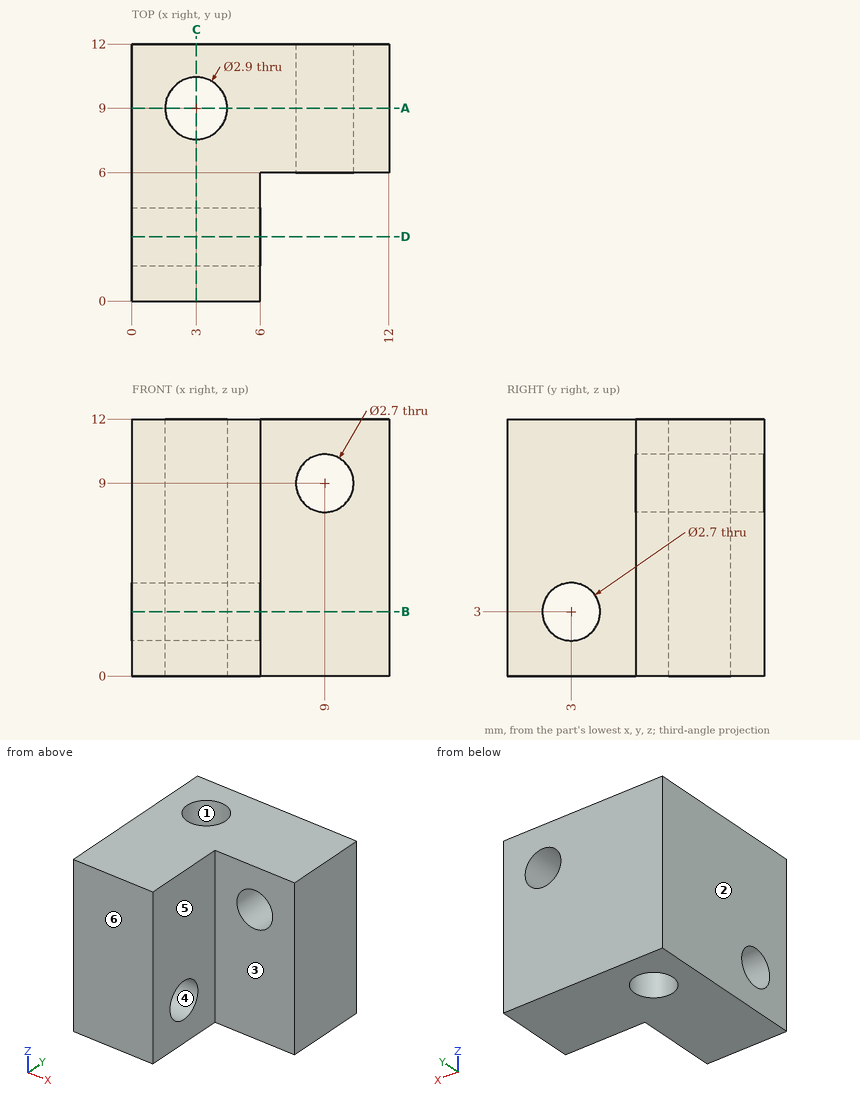
Geometry: see drawing. Coordinates: mm, zero at the bounding-box minimum. A direction names the side the tool comes from. Give positions to 0.01 mm unless a question says otherwise; leave off trailing zeros. Order: outer loops, then holes, each group sorted by start corner. A loop starts at its lowest first (then second) coordinate and runs counter-clockwise, first axis right, second up. Notation, with made-up numbers: (4.5, 77) -> (24.5, 77) arc R14 cw to (24.5, 99) -> close; hole circle Ø11 at (18, 4.5). An arc over 180 degrees is marked (long way). Write each question's results on one line, items separated by ' | '.
1) Cut plane A-A (y = 9). Output: boundary loops of the cut face in (x, z).
Geometry says:
outline: (0, 0) -> (1.55, 0) -> (1.55, 12) -> (0, 12) -> close; (4.45, 0) -> (12, 0) -> (12, 12) -> (4.45, 12) -> close; hole circle Ø2.7 at (9, 9)
2) Cut plane D-D (y = 3). Output: boundary loops of the cut face in (x, z), and give its area (3 significant figures).
Geometry says:
outline: (0, 0) -> (6, 0) -> (6, 1.65) -> (0, 1.65) -> close; (0, 4.35) -> (6, 4.35) -> (6, 12) -> (0, 12) -> close | area: 55.8 mm²
3) Cut plane C-C (x = 3). Output: boundary loops of the cut face in (y, z).
Geometry says:
outline: (0, 0) -> (7.55, 0) -> (7.55, 12) -> (0, 12) -> close; (10.45, 0) -> (12, 0) -> (12, 12) -> (10.45, 12) -> close; hole circle Ø2.7 at (3, 3)
4) Draft query along Y for the marked faces 1, 2, 3 and 4. Return one class per face: released by +Y, released by -Y, zero draft, split by the parting line, or undercut.
Geometry says:
face 1: undercut | face 2: zero draft | face 3: released by -Y | face 4: undercut
5) Set-up query: the marked faces 5 and 6. Return all of +Z, -Z, +X, -X, +Y, -Y with unobstructed straight access to the full face (end or side cutting, diameter ignored); none if empty.
Geometry says:
face 5: +Z, -Z, +X, -Y | face 6: +Z, -Z, +X, -X, -Y
6) Cut plane B-B (z = 3). Output: boundary loops of the cut face in (x, y), and give its area (3 significant figures).
Geometry says:
outline: (0, 0) -> (6, 0) -> (6, 1.65) -> (0, 1.65) -> close; (0, 4.35) -> (6, 4.35) -> (6, 6) -> (12, 6) -> (12, 12) -> (0, 12) -> close; hole circle Ø2.9 at (3, 9) | area: 85.2 mm²
7) Line query: line 1 along Y through (x, z) = (3, 3); line 2 along X through (y, z) = (8.75, 8.5); line 3 along X through (y, z) = (3.5, 11.75). Output: solid intervals per line, ascending.
Geometry says:
line 1: y = 0 to 1.65, 4.35 to 7.55, 10.45 to 12 | line 2: x = 0 to 1.57, 4.43 to 7.75, 10.25 to 12 | line 3: x = 0 to 6
8) First-contact query: pin 1 Ø4 at (x, z) = (8.5, 7.5) entering from -Y; pin 2 Ø4.5 at (y, z) = (3, 3) entering from +X; pin 3 Ø2 at (x, z) = (9, 9) entering from -Y. Flat tips, straight axial feed; report the tip coordinate or a pass-through.
Geometry says:
pin 1: stops at y = 6 | pin 2: stops at x = 6 | pin 3: passes through
